Input: part model. Units: mm. Frame: model coordinates. A direction names the side the tool comes from. Give positions to 0.01 mm unless a question says otherwise; leave off trailing zeros. Loops run counter-clockwise (first coordinate to the right, second up) from the corner with the lowest first, then second, coordinate; pieces in that order, holes last. Notation, with made-up numbers: (39.25, 54) - (46.25, 54) arc R22 ccw to (46.25, 75) - close; hole circle Ø1 at (89.5, 10). An arc over 180 degrees is marked (long way). Answer as a JSON object with one key per item and string values. Group by question number.
(1) Pin query (flat end, axial travel): P1, Ø2, axis at x = -41.5, z = 8.5, coming from the -Y side; P2, Ø4, axis at x = 11.5, y = 25.5, coming from the -Z side; P3, Ø1.5, axis at x = 8, y = 0, coming from the +Z side. Return the tip coordinate at first contact, or that it passes through.
(2) Section query D-D (y = 8). Return loops of the section in (x, z).
(3) Section query B-B (y = -35.5). Return loops of the section in (x, z).
(4) Access query for faces 1 (the flat face through (-2.465, -41.014, 133.409)), 2 (the flat face through (0.2, -40.2, 17)), 3 (the flat face through (-1, 40, 86)). Directions: +Z, -Z, +X, -X, +Y, -Y. A direction counts if a zero-diameter tool reaches every point of the face in a straight line with its end or side. Return the directions, or none.
(5) Section query C-C (z = 150). Return loops of the section in (x, y).
(6) Section query A-A (x = 19). Return loops of the section in (y, z), plus the area to 3 significant figures.
(7) Mould query, pull axis Y, two halves, no side actions, for faces 4 (the flat face through (40, -1, 86)), 5 (the flat face through (-10, -42, 91)), 6 (the flat face through (-3.3, -40.2, 167)). Classes: +Y half, -Y half, draft (parallel to the pull), parting line (faces both ways), or undercut.
(8) Material intervals for L1, parallel to X at y = 9, z = 88; L2, parallel to Y at x = -3, z = 116, sorted ascending.
```python
from build123d import *

# Parameters (mm, degrees)
F0_W     = 84
F0_H     = 84
F1_DEPTH = 167
F2_W     = 80
F2_H     = 80
F3_DEPTH = 165
F4_W     = 20
F4_H     = 15
F5_DEPTH = 84
F6_W     = 10
F6_H     = 80
F7_DEPTH = 2


with BuildPart() as f1:
    # F0 (on Top) → F1 (new body)
    with BuildSketch(Plane.XY):
        Rectangle(F0_W, F0_H)
    extrude(amount=F1_DEPTH)

    # F2 (on face) → F3 (cut)
    with BuildSketch(Plane.XY.offset(167)):
        Rectangle(F2_W, F2_H)
    extrude(amount=-F3_DEPTH, mode=Mode.SUBTRACT)

    # F4 (on face) → F5 (cut)
    with BuildSketch(Plane.YZ.offset(42)):
        with Locations((-32, 9.5)):
            Rectangle(F4_W, F4_H)
    extrude(amount=-F5_DEPTH, mode=Mode.SUBTRACT)

    # F6 (on face) → F7 (cut)
    with BuildSketch(Plane.XZ.offset(42)):
        Polygon((5, 49.017786), (-5, 49.017786), (0, 40.357532), align=None)
        with Locations((0, 89.017786)):
            Rectangle(F6_W, F6_H)
        Polygon((0, 137.67804), (-5, 129.017786), (5, 129.017786), align=None)
    extrude(amount=-F7_DEPTH, mode=Mode.SUBTRACT)


solid = f1.part
```
Recorded:
{
 "1": {"P1": "stops at y = -22", "P2": "stops at z = 0", "P3": "stops at z = 2"},
 "2": {"outline": "(-42, 0) - (42, 0) - (42, 167) - (40, 167) - (40, 2) - (-40, 2) - (-40, 167) - (-42, 167) - close"},
 "3": {"outline": "(-42, 0) - (42, 0) - (42, 2) - (-42, 2) - close; (-42, 17) - (-40, 17) - (-40, 167) - (-42, 167) - close; (40, 17) - (42, 17) - (42, 167) - (40, 167) - close"},
 "4": {"face 1": "-Y", "face 2": "+X, -X, -Y", "face 3": "+Z"},
 "5": {"outline": "(-42, -42) - (42, -42) - (42, 42) - (-42, 42) - close; hole (-40, -40) - (40, -40) - (40, 40) - (-40, 40) - close"},
 "6": {"outline": "(-42, 0) - (42, 0) - (42, 167) - (40, 167) - (40, 2) - (-42, 2) - close; (-42, 17) - (-40, 17) - (-40, 167) - (-42, 167) - close", "area": "798 mm^2"},
 "7": {"face 4": "undercut", "face 5": "-Y half", "face 6": "draft"},
 "8": {"L1": "x = -42 to -40, 40 to 42", "L2": "y = 40 to 42"}
}
